from build123d import *

# Parameters (mm, degrees)
SKETCH_1_W      = 3
SKETCH_1_H      = 10
SKETCH_1_W_2    = 5
SKETCH_1_H_2    = 3
EXTRUDE_1_DEPTH = 3


with BuildPart() as part:
    # 草圖1 → 填料-伸長1 (new body)
    with BuildSketch(Plane.XY):
        with Locations((-48.5, -4.734163056)):
            Rectangle(SKETCH_1_W, SKETCH_1_H)
        Polygon((-5, -27.234163056), (0, -27.234163056), (5, -27.234163056), (47, -27.234163056), (47, -9.734163056), (47, 0.265836944), (47, 10.265836944), (47, 20.265836944), (47, 25.265836944), (-47, 25.265836944), (-47, 20.265836944), (-47, 10.265836944), (-47, 0.265836944), (-47, -9.734163056), (-47, -27.234163056), align=None)
        with Locations((-2.5, -28.734163056)):
            Rectangle(SKETCH_1_W_2, SKETCH_1_H_2)
        with Locations((2.5, -28.734163056)):
            Rectangle(SKETCH_1_W_2, SKETCH_1_H_2)
        with Locations((-48.5, 15.265836944)):
            Rectangle(SKETCH_1_W, SKETCH_1_H)
        with Locations((48.5, 15.265836944)):
            Rectangle(SKETCH_1_W, SKETCH_1_H)
        with Locations((48.5, -4.734163056)):
            Rectangle(SKETCH_1_W, SKETCH_1_H)
    extrude(amount=EXTRUDE_1_DEPTH)


solid = part.part
Design review of the part built by this model. Coordinates are the model's own, in mm. A direction names the side the tool comes from. Round coordinates to 2 decimals unless told otherwise and drop trailing zeros. Write each loop counter-clockwise with the first axis right and the second up, starting at its lowest first coordinate (ties: lowest second). Pieces come first, ordered by that corner, then holes. Notation, with made-up numbers: M 13,-29.75 L 61,-29.75 A19 cw 61,-23.75 Z; hole C 0.5,-4 d11. An arc over 180 degrees is marked long. One line per item, written item: value. Start each with the question number.
1. To check wall thickness, follow probe 1 along Y at (x, z) = (9, 0.6); probe 2 along X at (y, z) = (-26.5, 0.2). State the ranges of each line that lie inside material, in increasing order. Write a range as from..to.
2. Take a section at B-B on x = -8. State the section outline as (y, z) points.
3. Draft analysis for pull direction Y (two halves, no side actions). For faces 4 (the face through (47, 5, 1)), 5 (the face through (-47, 23, 1)), 6 (the face through (48, -9.734, 1)), state which applies: pulls with the +Y half, pulls with the -Y half, needs draft (parallel to the pull), parting line crosses it, or undercut.
4. Clearance check with flat-ended pins moving along their axes: P1, Ø0.9, axis at x = 28, z = 1.5, coming from the -Y side; P2, Ø1.5, axis at x = 48.5, z = 2, coming from the -Y side; P3, Ø1.5, axis at y = 23.5, z = 1.5, coming from the -X side. State where each tip first meets the part, or that it passes through.
5. For faces 1 (the face through (48, 0.266, 1)), 2 (the face through (-5, -29, 1)), 3 (the face through (-49, 0.266, 1)), list the 3-axis set-ups (+Z, -Z, +X, -X, +Y, -Y) from which the entire face can be reached by the end or side of a thin tool; tool diameter is ignored.
6. Take a section at C-C on y = -14. State the section outline as (x, z) points, then the cut area to 3 significant figures.
7. Take a section at A-A on z = 1. State the section outline as (x, y) points.
Computed:
1. probe 1: y = -27.23..25.27
1. probe 2: x = -47..47
2. outline: M -27.23,0 L 25.27,0 L 25.27,3 L -27.23,3 Z
3. face 4: undercut
3. face 5: needs draft
3. face 6: pulls with the -Y half
4. P1: stops at y = -27.23
4. P2: stops at y = -9.73
4. P3: stops at x = -47
5. face 1: +Z, -Z, +X
5. face 2: +Z, -Z, -X, -Y
5. face 3: +Z, -Z, -X
6. outline: M -47,0 L 47,0 L 47,3 L -47,3 Z
6. area: 282 mm²
7. outline: M -50,-9.73 L -47,-9.73 L -47,-27.23 L -5,-27.23 L -5,-30.23 L 5,-30.23 L 5,-27.23 L 47,-27.23 L 47,-9.73 L 50,-9.73 L 50,0.27 L 47,0.27 L 47,10.27 L 50,10.27 L 50,20.27 L 47,20.27 L 47,25.27 L -47,25.27 L -47,20.27 L -50,20.27 L -50,10.27 L -47,10.27 L -47,0.27 L -50,0.27 Z
